from build123d import *

# Parameters (mm, degrees)
BOSS_EXTRUDE1_DEPTH   = 15
F_8_0MM_DOWEL_HOLE1_D = 8


with BuildPart() as part:
    # Sketch1 → Boss-Extrude1 (new body)
    with BuildSketch(Plane.XY):
        with BuildLine():
            Line((9.905, 0), (-9.905, 0))
            ThreePointArc((-9.905, 0), (-10.046421356, -0.058578644), (-10.105, -0.2))
            Line((-10.105, -0.2), (-10.105, -1.2))
            ThreePointArc((-10.105, -1.2), (-9.519213562, -2.614213562), (-8.105, -3.2))
            Line((-8.105, -3.2), (8.105, -3.2))
            ThreePointArc((8.105, -3.2), (9.519213562, -2.614213562), (10.105, -1.2))
            Line((10.105, -1.2), (10.105, -0.2))
            ThreePointArc((10.105, -0.2), (10.046421356, -0.058578644), (9.905, 0))
        make_face()
    extrude(amount=BOSS_EXTRUDE1_DEPTH)

    # Ø8.0mm Dowel Hole1 (through all)
    with Locations(Plane(origin=(0, 0, 0), x_dir=(1, 0, 0), z_dir=(0, 1, 0))):
        with Locations((0, -7.5)):
            Hole(F_8_0MM_DOWEL_HOLE1_D / 2)


solid = part.part
Work out the finished part from the listing and answer in its coordinate system (mm). Coordinates: 2 decimals unless noted, no trailing zeros. Write each loop counter-clockwise with the first axis right and the second up, starting at its lowest first coordinate (ties: lowest second). Pieces come first, ordered by that corner, then holes. Notation, with made-up numbers: M 1.25,-1.75 L 6.25,-1.75 A17 cw 6.25,28.25 Z; hole C 42,-17.75 d8. An arc over 180 degrees is marked long. Use one line per item in the form item = value. Start each with the question number.
1. The part is cut by section D-D (y = -1.7). Give the vertices of the cut face in (x, z).
2. The part is cut by section C-C (z = 2.5). Give the vertices of the cut face in (x, y) (3 decimals), plus the area to 3 significant figures.
3. Each of these flat-tipped pins is pushed along its axis until it touches: P1, Ø1, axis at y = -3, z = 7.5, coming from the +X side; P2, Ø1, axis at y = -3, z = 6, coming from the -X side. Where does it stop, or does it pass through?
4. Straight lines are drawn through the part: probe 1 along Z at (x, y) = (0, -1.15); probe 2 along Z at (x, y) = (1.5, -3); probe 3 along X at (y, z) = (-2.9, 4.75). For each, find the intervals that lie inside material, in ascending order. Write a range as from..to.
5. The part is cut by section B-B (x = 0). Give the vertices of the cut face in (y, z), plus the area to 3 significant figures.
6. The mould has two halves that part along Z. Classify faces 1 (the face through (0, -2, 15)), 2 (the face through (-9.535, -2.599, 7.395)), 3 (the face through (-3.815, -1.622, 6.299)), 4 (the face through (0, -2, 0)): released by +Z, released by -Z, zero draft, split by the parting line, or undercut.
7. The part is cut by section A-A (z = 7.5). Give the vertices of the cut face in (x, y) (3 decimals), plus the area to 3 significant figures.
Evaluation:
q1.outline = M -10.04,0 L 10.04,0 L 10.04,15 L -10.04,15 Z; hole C 0,7.5 d8
q2.outline = M -10.105,-1.2 A2 ccw -8.105,-3.2 L 8.105,-3.2 A2 ccw 10.105,-1.2 L 10.105,-0.2 A0.2 ccw 9.905,0 L -9.905,0 A0.2 ccw -10.105,-0.2 Z
q2.area = 62.9 mm^2
q3.P1 = 9.62
q3.P2 = -9.62
q4.probe_1 = 0..3.5, 11.5..15
q4.probe_2 = 0..3.79, 11.21..15
q4.probe_3 = -9.16..-2.9, 2.9..9.16
q5.outline = M -3.2,0 L 0,0 L 0,3.5 L -3.2,3.5 Z; M -3.2,11.5 L 0,11.5 L 0,15 L -3.2,15 Z
q5.area = 22.4 mm^2
q6.face_1 = released by +Z
q6.face_2 = zero draft
q6.face_3 = undercut
q6.face_4 = released by -Z
q7.outline = M -10.105,-1.2 A2 ccw -8.105,-3.2 L -4,-3.2 L -4,0 L -9.905,0 A0.2 ccw -10.105,-0.2 Z; M 4,-3.2 L 8.105,-3.2 A2 ccw 10.105,-1.2 L 10.105,-0.2 A0.2 ccw 9.905,0 L 4,0 Z
q7.area = 37.3 mm^2
